```python
from build123d import *

# Parameters (mm, degrees)
F0_W     = 45.25
F0_H     = 26
F0_W_2   = 25
F0_H_2   = 24
F0_R     = 1
F0_R_2   = 8.5
F1_DEPTH = 2
F3_DEPTH = 2
F4_R     = 1
F5_DEPTH = 2
F6_SIZE  = 8.5
F7_R     = 1
F7_R_2   = 0.99999


# Not quite as in the source:
# - a fillet or chamfer is up to 0.001 mm smaller than in the source, because OpenCascade refuses the exact size


with BuildPart() as f1:
    # F0 (on Front) → F1 (new body)
    with BuildSketch(Plane.XZ):
        Rectangle(F0_W, F0_H)
        Rectangle(F0_W_2, F0_H_2, mode=Mode.SUBTRACT)
        Rectangle(F0_W_2, F0_H_2)
        with Locations((-10.5, -10)):
            Circle(F0_R, mode=Mode.SUBTRACT)
        with Locations((10.5, -10)):
            Circle(F0_R, mode=Mode.SUBTRACT)
        with Locations((-10.5, 2.5)):
            Circle(F0_R, mode=Mode.SUBTRACT)
        Circle(F0_R_2, mode=Mode.SUBTRACT)
        with Locations((10.5, 2.5)):
            Circle(F0_R, mode=Mode.SUBTRACT)
    extrude(amount=-F1_DEPTH)

    # F2 (on face) → F3 (join)
    with BuildSketch(Plane.YZ.offset(22.625)):
        with BuildLine():
            ThreePointArc((20, -4.4), (15.6, 0), (20, 4.4))
            Line((20, 4.4), (2, 4.4))
            Line((2, 4.4), (2, -4.4))
            Line((2, -4.4), (20, -4.4))
        make_face()
        with BuildLine():
            ThreePointArc((20, 1.5), (21.0606601718, 1.0606601718), (21.5, 0))
            ThreePointArc((21.5, 0), (21.0606601718, -1.0606601718), (20, -1.5))
            Line((20, -1.5), (20, -4.4))
            ThreePointArc((20, -4.4), (23.1112698372, -3.1112698372), (24.4, 0))
            ThreePointArc((24.4, 0), (23.1112698372, 3.1112698372), (20, 4.4))
            Line((20, 4.4), (20, 1.5))
        make_face()
        with BuildLine():
            ThreePointArc((20, -1.5), (18.5, 0), (20, 1.5))
            Line((20, 1.5), (20, 4.4))
            ThreePointArc((20, 4.4), (15.6, 0), (20, -4.4))
            Line((20, -4.4), (20, -1.5))
        make_face()
    extrude(amount=-F3_DEPTH)

    # F4 (on face) → F5 (join)
    with BuildSketch(Plane(origin=(-22.625, 0, 0), x_dir=(0, -1, 0), z_dir=(-1, 0, 0))):
        with BuildLine():
            ThreePointArc((-20, -2.375), (-22.375, 0), (-20, 2.375))
            Line((-20, 2.375), (-20, 4.4))
            ThreePointArc((-20, 4.4), (-24.4, 0), (-20, -4.4))
            Line((-20, -4.4), (-20, -2.375))
        make_face()
        with BuildLine():
            ThreePointArc((-20, 2.375), (-18.3206213947, 1.6793786053), (-17.625, 0))
            ThreePointArc((-17.625, 0), (-18.3206213947, -1.6793786053), (-20, -2.375))
            Line((-20, -2.375), (-20, -4.4))
            ThreePointArc((-20, -4.4), (-16.8887301628, -3.1112698372), (-15.6, 0))
            ThreePointArc((-15.6, 0), (-16.8887301628, 3.1112698372), (-20, 4.4))
            Line((-20, 4.4), (-20, 2.375))
        make_face()
        with BuildLine():
            Line((-2, 4.4), (-20, 4.4))
            ThreePointArc((-20, 4.4), (-16.8887301628, 3.1112698372), (-15.6, 0))
            ThreePointArc((-15.6, 0), (-16.8887301628, -3.1112698372), (-20, -4.4))
            Line((-20, -4.4), (-2, -4.4))
            Line((-2, -4.4), (-2, 4.4))
        make_face()
        with Locations((-13.33, 0)):
            Circle(F4_R, mode=Mode.SUBTRACT)
        with Locations((-7.33, 0)):
            Circle(F4_R, mode=Mode.SUBTRACT)
    extrude(amount=-F5_DEPTH)

    # F6
    f6_edges = [f1.edges().sort_by_distance(p)[0] for p in [
        (22.625, 1, 13),
        (-22.625, 1, 13),
        (-22.625, 1, -13),
        (22.625, 1, -13),
    ]]
    chamfer(f6_edges, length=F6_SIZE)

    # F7 (call 1 of 10: OpenCascade refuses the feature's edges together)
    f7_edges = [f1.edges().sort_by_distance(p)[0] for p in [
        (-8.5, 2, 0),
    ]]
    fillet(f7_edges, radius=F7_R)

    # F7#2 (call 2 of 10)
    f7_2_edges = [f1.edges().sort_by_distance(p)[0] for p in [
        (18.375, 0, 8.75),
        (18.375, 0, -8.75),
        (22.625, 0, 0),
    ]]
    fillet(f7_2_edges, radius=F7_R)

    # F7#3 (call 3 of 10)
    f7_3_edges = [f1.edges().sort_by_distance(p)[0] for p in [
        (-18.375, 0, -8.75),
    ]]
    fillet(f7_3_edges, radius=F7_R)

    # F7#4 (call 4 of 10)
    f7_4_edges = [f1.edges().sort_by_distance(p)[0] for p in [
        (-18.375, 0, 8.75),
    ]]
    fillet(f7_4_edges, radius=F7_R)

    # F7#5 (call 5 of 10)
    f7_5_edges = [f1.edges().sort_by_distance(p)[0] for p in [
        (-22.625, 11, -4.4),
    ]]
    fillet(f7_5_edges, radius=F7_R)

    # F7#6 (call 6 of 10)
    f7_6_edges = [f1.edges().sort_by_distance(p)[0] for p in [
        (22.625, 11, 4.4),
    ]]
    fillet(f7_6_edges, radius=F7_R)

    # F7#7 (call 7 of 10)
    f7_7_edges = [f1.edges().sort_by_distance(p)[0] for p in [
        (0, 2, -13),
    ]]
    fillet(f7_7_edges, radius=F7_R)

    # F7#8 (call 8 of 10)
    f7_8_edges = [f1.edges().sort_by_distance(p)[0] for p in [
        (0, 2, 13),
    ]]
    fillet(f7_8_edges, radius=F7_R)

    # F7#9 (call 9 of 10) (radius 1 in the source; OpenCascade refuses exactly that, so slightly less here)
    f7_9_edges = [f1.edges().sort_by_distance(p)[0] for p in [
        (-20.625, 11, 4.4),
    ]]
    fillet(f7_9_edges, radius=F7_R_2)

    # F7#10 (call 10 of 10) (radius 1 in the source; OpenCascade refuses exactly that, so slightly less here)
    f7_10_edges = [f1.edges().sort_by_distance(p)[0] for p in [
        (20.625, 11, 4.4),
    ]]
    fillet(f7_10_edges, radius=F7_R_2)


solid = f1.part
```
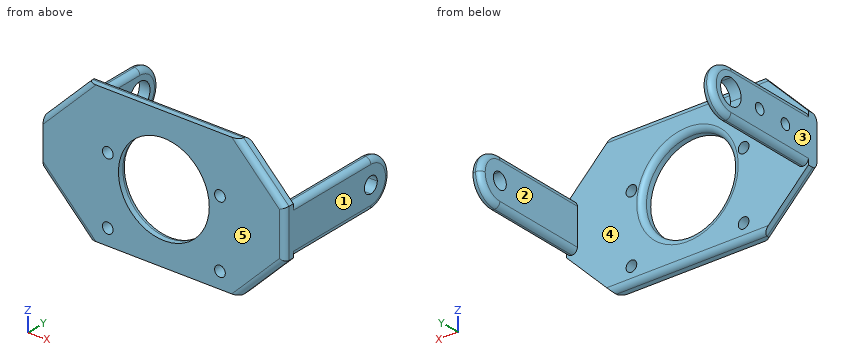
Here's how the part is built. I have some questions about the finished solid (model axes, mm). Face numbers are marked on the shaded views. A direction names the side the tool comes from. Round coordinates to 2 decimals unless told otherwise and drop trailing zeros. Order: outer loops, then holes, each group sorted by start corner. A loop starts at its lowest first (then second) coordinate and runs counter-clockwise, first axis right, second up. Notation, with made-up numbers: M 53,50 L 58,50 A16 cw 58,54 Z; hole C 29.5,33 d4. An arc over 180 degrees is marked long. Answer in a Markdown table with one row per item.
Item 1: Thinking about a two-plate mould opening in X: for the marked faces 3, 4 and 5, which applies, +X half, -X half, draft (parallel to the pull), parting line (faces both ways), or undercut?
A:
| item | result |
|---|---|
| face 3 | -X half |
| face 4 | undercut |
| face 5 | draft |
Item 2: If I drill on L1, parallel to Z at x = -10.5, y = 0.55; L2, parallel to X at y = 11.75, z = 3.25 (3 decimals); L3, parallel to Z at x = 0, y = 0.4, over which ranges is the centre line in solid material (lowest first)? Write a range as from..to.
A:
| item | result |
|---|---|
| L1 | z = -13..-11, -9..1.5, 3.5..13 |
| L2 | x = -22.625..-20.625, 20.625..22.625 |
| L3 | z = -13..-8.5, 8.5..13 |
Item 3: Imagine slicing it at D-D, the plane z = -10. State how many separate pieces and enclosed holes the cut face has, and give its area (3 significant figures).
A:
| item | result |
|---|---|
| separate pieces | 3 |
| enclosed holes | 0 |
| area | 59.9 mm2 |
Item 4: I'm going to push flat-ended pins straight in: pin 1 (2.5 mm diameter, centred on x = -10.5, z = -10, fed in from -Y); pin 2 (2.5 mm diameter, centred on x = -10.5, z = 2.5, fed in from +Y). Where does each tip first touch, or does it pass through?
A:
| item | result |
|---|---|
| pin 1 | stops at y = 0 |
| pin 2 | stops at y = 2 |
Item 5: For the marked faces 1 and 2, which set-ups out of +Z, -Z, +X, -X, +Y, -Y let a thin tool reach every point of the face, with its end or its side?
A:
| item | result |
|---|---|
| face 1 | +Z, -Z, +X, +Y, -Y |
| face 2 | +Z, -Z, +Y |
Item 6: Imagine slicing it at A-A, the plane x = 10.5. Write out the boundary of the cut face in (y, z).
A:
| item | result |
|---|---|
| outline | M 0,-13 L 1,-13 A1 ccw 2,-12 L 2,-11 L 0,-11 Z; M 0,-9 L 2,-9 L 2,1.5 L 0,1.5 Z; M 0,3.5 L 2,3.5 L 2,12 A1 ccw 1,13 L 0,13 Z |
Item 7: Imagine slicing it at C-C, the plane x = 0. Write out the boundary of the cut face in (y, z), and give its area (3 significant figures).
A:
| item | result |
|---|---|
| outline | M 0,-13 L 1,-13 A1 ccw 2,-12 L 2,-9.5 A1 ccw 1,-8.5 L 0,-8.5 Z; M 0,8.5 L 1,8.5 A1 ccw 2,9.5 L 2,12 A1 ccw 1,13 L 0,13 Z |
| area | 17.1 mm2 |
